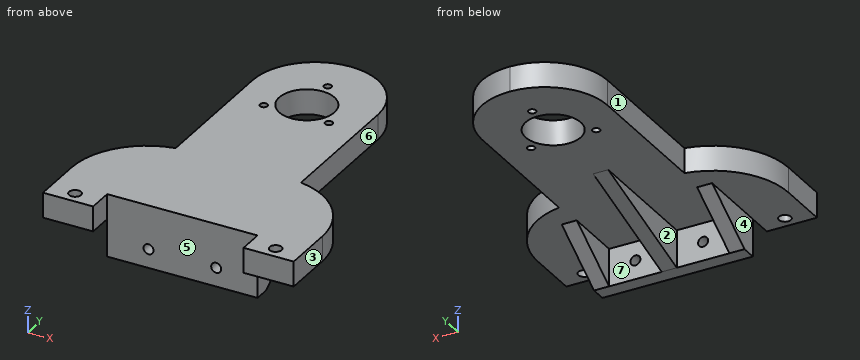
```python
from build123d import *

# Parameters (mm, degrees)
SKETCH2_W           = 100
SKETCH2_H           = 130
BOSS_EXTRUDE1_DEPTH = 10
SKETCH4_W           = 60
SKETCH4_H           = 10
SKETCH4_W_2         = 25
SKETCH4_H_2         = 80
CUT_EXTRUDE1_DEPTH  = 55
SKETCH6_W           = 60
SKETCH6_H           = 6
BOSS_EXTRUDE2_DEPTH = 15
SKETCH10_R          = 2.4
CUT_EXTRUDE3_DEPTH  = 15
FILLET6_R           = 30
FILLET7_R           = 30
RIB9_REACH          = 85.367
SKETCH12_WALL_W     = 219.977831906
SKETCH12_WALL_H     = 6
RIB10_START         = -6
RIB10_DEPTH         = 6
SKETCH14_R          = 2
CUT_EXTRUDE4_DEPTH  = 15
FILLET8_R           = 25
SKETCH15_R          = 11
CUT_EXTRUDE5_DEPTH  = 15
SKETCH17_R          = 1.5
CUT_EXTRUDE6_DEPTH  = 15


# Read off the part's stored shape, not the designer's step: Rib10
# Some blends are built 0.0001 mm under size
with BuildPart() as part:
    # Sketch2 → Boss-Extrude1 (new body)
    with BuildSketch(Plane.XY):
        Rectangle(SKETCH2_W, SKETCH2_H)
    extrude(amount=BOSS_EXTRUDE1_DEPTH)

    # Sketch4 → Cut-Extrude1 (cut)
    with BuildSketch(Plane.XY.offset(10)):
        with Locations((0, -60)):
            Rectangle(SKETCH4_W, SKETCH4_H)
        with Locations((-37.5, 25)):
            Rectangle(SKETCH4_W_2, SKETCH4_H_2)
        with Locations((37.5, 25)):
            Rectangle(SKETCH4_W_2, SKETCH4_H_2)
    extrude(amount=-CUT_EXTRUDE1_DEPTH, mode=Mode.SUBTRACT)

    # Sketch6 → Boss-Extrude2 (add)
    with BuildSketch(Plane(origin=(0, 0, 0), x_dir=(-1, 0, 0), z_dir=(0, 0, -1))):
        with Locations((0, -52)):
            Rectangle(SKETCH6_W, SKETCH6_H)
    extrude(amount=BOSS_EXTRUDE2_DEPTH)

    # Sketch10 → Cut-Extrude3 (cut)
    with BuildSketch(Plane.XY.offset(10)):
        with Locations((-40, -60)):
            Circle(SKETCH10_R)
        with Locations((40, -60)):
            Circle(SKETCH10_R)
    extrude(amount=-CUT_EXTRUDE3_DEPTH, mode=Mode.SUBTRACT)

    # Fillet6
    # the kernel refuses this fillet: 30 mm, written as the material it takes off along each edge
    with BuildSketch(Plane(origin=(50, -15, 83.950997289), x_dir=(-1, 0, 0), z_dir=(0, 0, -1))) as fillet6_piece_1:
        with BuildLine():
            CenterArc((30, -29.580398915), FILLET6_R, 99.594068227, 80.405931773)
            Line((0, -29.580398916), (-0.6, -29.580398916))
            Line((-0.6, -29.580398916), (-0.6, 0))
            Line((-0.6, 0), (0, 0.6))
            ThreePointArc((0, 0.6), (12.5, 0.6), (24.9, 0.591607978))
            Line((24.9, 0.591607978), (25, 0))
        make_face()
    extrude(amount=157.901994578, mode=Mode.SUBTRACT)

    # Fillet7
    # the kernel refuses this fillet: 30 mm, written as the material it takes off along each edge
    with BuildSketch(Plane(origin=(-50, -15, 83.950997289), x_dir=(0, -1, 0), z_dir=(0, 0, -1))) as fillet7_piece_1:
        with BuildLine():
            CenterArc((29.580398916, -30), FILLET7_R, 90, 80.405931773)
            Line((0, -25), (-0.591607978, -24.9))
            ThreePointArc((-0.591607978, -24.9), (-0.6, -12.5), (-0.6, 0))
            Line((-0.6, 0), (0, 0.6))
            Line((0, 0.6), (29.580398916, 0.6))
            Line((29.580398916, 0.6), (29.580398916, 0))
        make_face()
    extrude(amount=157.901994578, mode=Mode.SUBTRACT)

    # Sketch12 wall → Rib9 (add, up to next)
    with BuildSketch(Plane(origin=(0, -24.5, -7.5), x_dir=(0, 0.956199955507, 0.292714272094), z_dir=(0, -0.292714272094, 0.956199955507)), mode=Mode.PRIVATE) as rib9_sk1:
        Rectangle(SKETCH12_WALL_W, SKETCH12_WALL_H)
    rib9_tool1 = extrude(rib9_sk1.sketch, amount=RIB9_REACH, mode=Mode.PRIVATE) - part.part
    add(rib9_tool1.solids().sort_by_distance((0, -24.5, -7.5))[0])

    # Rib10 outline → Rib10 (add)
    with BuildSketch(Plane.ZY.offset(30).offset(RIB10_START)):
        Polygon((0, -25.879609738), (-15, -49), (0, -49), align=None)
    rib10 = extrude(amount=RIB10_DEPTH)

    # Mirror4: Rib10 across plane
    add(rib10.mirror(Plane(origin=(0, 0, 0), x_dir=(0, 0, 1), z_dir=(1, 0, 0))))

    # Sketch14 → Cut-Extrude4 (cut)
    with BuildSketch(Plane(origin=(0, -49, 0), x_dir=(1, 0, 0), z_dir=(0, 1, 0))):
        with Locations(Location((-13.5, 7.5, 0), (0, 0, 270))):
            Circle(SKETCH14_R)
        with Locations(Location((13.5, 7.5, 0), (0, 0, 270))):
            Circle(SKETCH14_R)
    extrude(amount=-CUT_EXTRUDE4_DEPTH, mode=Mode.SUBTRACT)

    # Fillet8
    fillet8_edges = [part.edges().sort_by_distance(p)[0] for p in [
        (25, 65, 5),
        (-25, 65, 5),
    ]]
    fillet(fillet8_edges, radius=FILLET8_R - 0.0001)  # a hair under: the kernel refuses the full size

    # Sketch15 → Cut-Extrude5 (cut)
    with BuildSketch(Plane.XY.offset(10)):
        with Locations((0, 34)):
            Circle(SKETCH15_R)
    extrude(amount=-CUT_EXTRUDE5_DEPTH, mode=Mode.SUBTRACT)

    # Sketch17 → Cut-Extrude6 (cut)
    with BuildSketch(Plane.XY.offset(10)):
        with Locations((0, 49)):
            Circle(SKETCH17_R)
        with Locations((12.990381057, 26.5)):
            Circle(SKETCH17_R)
        with Locations((-12.990381057, 26.5)):
            Circle(SKETCH17_R)
    extrude(amount=-CUT_EXTRUDE6_DEPTH, mode=Mode.SUBTRACT)


solid = part.part
```
Verification items for the finished model (mm, model axes). Face numbers are marked on the shaded views. A direction names the side the tool comes from. Coordinates: 2 decimals unless noted, no trailing zeros. Write each loop counter-clockwise with the first axis right and the second up, starting at its lowest first coordinate (ties: lowest second). Pieces come first, ordered by that corner, then holes. Notation, with made-up numbers: M 61.5,12.5 L 112.5,12.5 A12 ccw 112.5,34.5 Z; hole C 42.25,60 d9. An arc over 180 degrees is marked long. Answer as a JSON object with one key per item and string values. Group by question number.
(1) Cross-section at C-C, the plane x = 5.5. Record the cut outline in (y, z), and give its area (3 significant figures).
(2) Gauge pin test, flat ends, axial feed: pin 1 (12 mm diameter, centred on y = -35.5, z = -7.5, fed in from +X); pin 2 (3 mm diameter, centred on y = -0.5, z = 6, fed in from +X); pin 3 (7.5 mm diameter, centred on y = -35.5, z = -4.5, fed in from -X). Record the tip position at first contact, or that the pin passes through.
(3) Tool access check on the marked faces 4, 5, 6 and 7. Record the directions out of +Z, -Z, +X, -X, +Y, -Y that give a thin tool (end or side, any length) a straight path to the whole face; none if there is none.
(4) Cross-section at D-D, the plane y = 49. Record the cut outline in (x, z), and give its area (3 significant figures).
(5) Cross-section at A-A, the plane y = -60. Record the cut outline in (x, z), and give its area (3 significant figures).
(6) Release check for a two-part mould opening along X. For the marked faces 1, 2 and 3 record: +X half, -X half, draft (parallel to the pull), parting line (faces both ways), or undercut.
(7) Material ranges on line 1 (Y direction, x = 0, z = 7); line 2 (X direction, y = -39.5, z = -5); line 3 (Y direction, x = 23.5, z = -0.5), recorded low to high.
(8) Cross-section at B-B, the plane z = 2. State how many separate pieces and enclosed holes the cut face has, and give its area (3 significant figures).
Reply:
{
 "1": {"outline": "M -55,-15 L -49,-15 L -49,0 L 24.47,0 L 24.47,10 L -55,10 Z; M 43.53,0 L 64.39,0 L 64.39,10 L 43.53,10 Z", "area": "1,090 mm²"},
 "2": {"pin 1": "x = 30", "pin 2": "x = 25", "pin 3": "x = -30"},
 "3": {"face 4": "-Z, -X, +Y, -Y", "face 5": "+Z, -Z, -Y", "face 6": "+Z, -Z, +X, +Y", "face 7": "-Z, +Y"},
 "4": {"outline": "M -23.32,0 L -1.5,0 L -1.5,10 L -23.32,10 Z; M 1.5,0 L 23.32,0 L 23.32,10 L 1.5,10 Z", "area": "436 mm²"},
 "5": {"outline": "M -50,0 L -42.4,0 L -42.4,10 L -50,10 Z; M -37.6,0 L -30,0 L -30,10 L -37.6,10 Z; M 30,0 L 37.6,0 L 37.6,10 L 30,10 Z; M 42.4,0 L 50,0 L 50,10 L 42.4,10 Z", "area": "304 mm²"},
 "6": {"face 1": "-X half", "face 2": "undercut", "face 3": "+X half"},
 "7": {"line 1": "-55 to 23, 45 to 47.5, 50.5 to 65", "line 2": "-30 to -24, -3 to 3, 24 to 30", "line 3": "-55 to -49"},
 "8": {"separate pieces": "1", "enclosed holes": "6", "area": "7,330 mm²"}
}
